Can you work these out from the drawing? Everything is in mm from the part's minimum corner. Round coordinates to 2 decimals unless told otherwise and drop trailing zeros. Write each loop counter-clockwise with the first axis right and the second up, starting at its lowest first coordinate (ties: lowest second). Pieces come first, ordered by that corner, then holes. Notation, with made-up numbers: M -16.75,32 L 6.25,32 A7 cw 6.25,43 Z; hole C -1.5,58.25 d10. An arc over 180 degrees is marked long. Use one line per item in the form item = value. Start each with the question number.
Q1. I'm going to push flat-ended pins straight in: pin 1 Ø0.9 at (x, z) = (1.5, 17.5) entering from +Y; pin 2 Ø0.9 at (x, z) = (1.5, 17) entering from -Y; pin 3 Ø1.5 at (x, y) = (1, 1.5) entering from -Z. Where does each tip first touch, or does it pass through?
Q2. I need wall thicknesses on line 1 along Y through (x, z) = (1, 66); line 2 along Z through (x, y) = (0.5, 34). Which ranges of each line are inside material? Lowest first, please. Write a range as from..to.
Q3. I want a section at A-A on x = 1.05. List the corners of the cut face in (y, z) for me.
Q4. I want a section at B-B on z = 17. List the corners of the cut face in (x, y) for me, and give its area (3 significant figures).
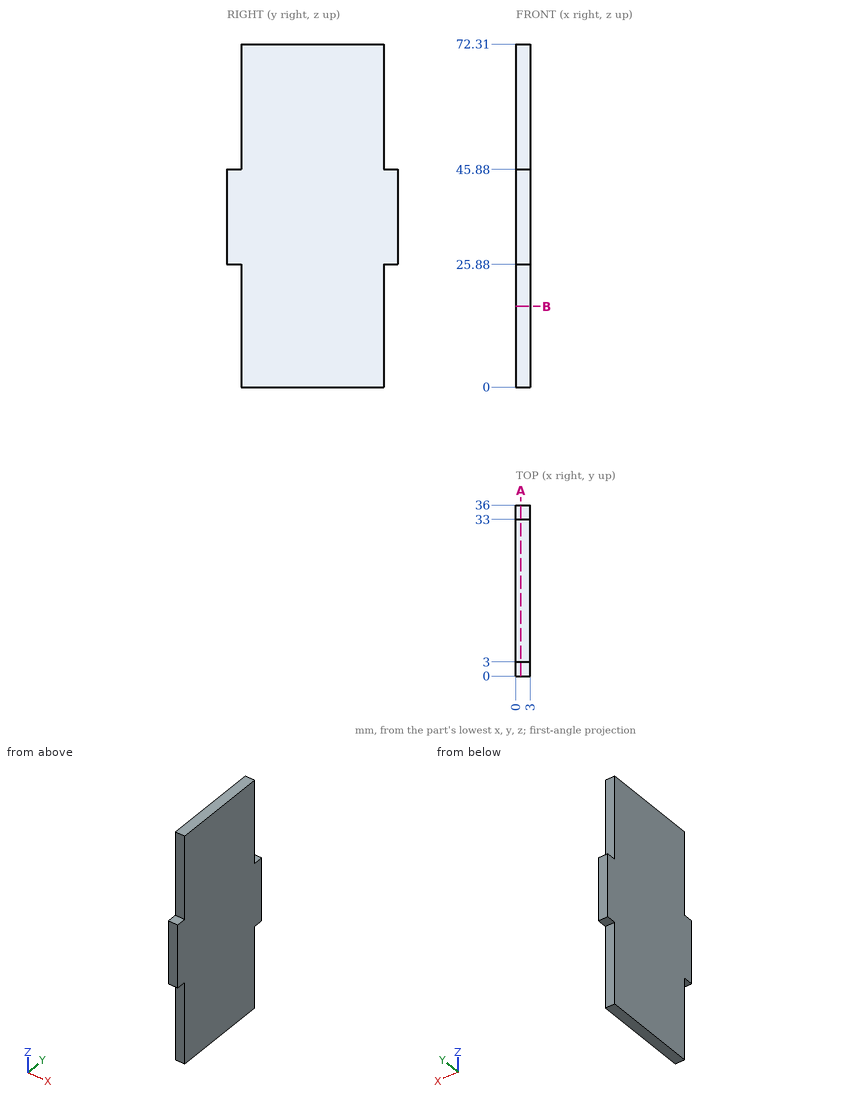
Reported:
q1.pin_1 = 33
q1.pin_2 = 3
q1.pin_3 = 25.88
q2.line_1 = 3..33
q2.line_2 = 25.88..45.88
q3.outline = M 0,25.88 L 3,25.88 L 3,0 L 33,0 L 33,25.88 L 36,25.88 L 36,45.88 L 33,45.88 L 33,72.31 L 3,72.31 L 3,45.88 L 0,45.88 Z
q4.outline = M 0,3 L 3,3 L 3,33 L 0,33 Z
q4.area = 90.0 mm^2
